Autodesk Fusion 360 part; units mm, degrees
sketch "Sketch1" plane through (0, 0, 0) normal (0, 0, 1) x (1, 0, 0)
  line L0 (13, -20) -> (-13, -20)
  line L1 (-13, -20) -> (-13, 20)
  line L2 (-13, 20) -> (13, 20)
  line L3 (13, 20) -> (13, -20)
  line L4 (13, -20) -> (-13, 20) construction
  line L5 (-13, -20) -> (13, 20) construction
  line L6 (0, 20) -> (0, -20)
  circle A0 centre (0, -4) radius 7
  circle A1 centre (0, 10) radius 1.7
  circle A2 centre (0, 10) radius 3
  line L7 (-3.85, 20) -> (-3.85, -20)
  line L8 (3.85, 20) -> (3.85, -20)
  circle A3 centre (0, -4) radius 1.7
  circle A4 centre (0, -4) radius 2.3
  line L9 (-3.85, 15) -> (3.85, 15)
  line L10 (-3.85, 5) -> (3.85, 5)
  line L11 (-3.85, -12) -> (3.85, -12)
  dimension "d1" = 26
  dimension "d2" = 40
  dimension "d3" = 14
  dimension "d4" = 16
  dimension "d5" = 3.4
  dimension "d6" = 6
  dimension "d7" = 7.7
  dimension "d8" = 10
  dimension "d9" = 3.4
  dimension "d10" = 4.6
  dimension "d15" = 5
  dimension "d16" = 5
  dimension "d17" = 8
extrude "Extrude1" add sketch "Sketch1" along normal blind 5 contours L0 L2 L3 A0 L8 | L0 L6 L8 L11 | L0 L6 L7 L11 | L6 A0 L8 L11 | L2 L6 L8 L9 | L0 L1 L2 A0 L7 | L6 A0 L7 L11 | A0 L8 | L6 A0 L8 A4 | L2 L6 L7 L9 | L6 A2 L8 L9 L10 | L6 A0 L7 A4 | L6 A0 L8 L10 | L6 A2 L7 L9 L10 | A0 L7 | L6 A3 A4 | L6 A3 A4 | L6 A0 L7 L10 | L6 A1 A2 | L6 A1 A2
extrude "Extrude13" cut sketch "Sketch1" along normal blind 10 contours L6 A3 | L6 A3 | L6 A1 | L6 A1
extrude "Extrude2" add sketch "Sketch1" along normal blind 0.8 from surface at 5 contours L0 L6 L8 L11 | L0 L6 L7 L11 | L2 L6 L8 L9 | L2 L6 L7 L9
fillet "Fillet1" radius 1 8 edges at (-3.85, 20, 5.4) (-3.85, 15, 5.4) (-3.85, -12, 5.4) (-3.85, -20, 5.4) (3.85, -12, 5.4) (3.85, -20, 5.4) (3.85, 15, 5.4) (3.85, 20, 5.4)
chamfer "Chamfer1" distance 0.2 angle 45 16 edges at (3.5571, 15.2929, 5.8) (0, 15, 5.8) (-3.5571, 15.2929, 5.8) (-3.85, 17.5, 5.8) (-3.5571, 19.7071, 5.8) (0, 20, 5.8) (3.5571, 19.7071, 5.8) (3.85, 17.5, 5.8) (3.5571, -19.7071, 5.8) (0, -20, 5.8) (-3.5571, -19.7071, 5.8) (-3.85, -16, 5.8) (-3.5571, -12.2929, 5.8) (0, -12, 5.8) (3.5571, -12.2929, 5.8) (3.85, -16, 5.8)
extrude "Extrude3" cut sketch "Sketch1" along normal blind 3 contours L6 A1 A2 | L6 A1 A2 | L6 A1 | L6 A1
extrude "Extrude5" cut sketch "Sketch1" against normal blind 5 from surface at 5 contours L6 A3 A4 | L6 A3 A4
chamfer "Chamfer3" distance 4 angle 45 4 edges at (13, -20, 2.5) (-13, -20, 2.5) (-13, 20, 2.5) (13, 20, 2.5)
fillet "Fillet2" radius 2 8 edges at (9, -20, 2.5) (-13, 16, 2.5) (13, -16, 2.5) (13, 16, 2.5) (9, 20, 2.5) (-9, 20, 2.5) (-13, -16, 2.5) (-9, -20, 2.5)
chamfer "Chamfer4" distance 0.2 angle 45 20 edges at (-2.1444, -3.1683, 5) (11, 18, 5) (8.9369, 19.8478, 5) (5.5108, 20, 5) (5.5108, -20, 5) (8.9369, -19.8478, 5) (11, -18, 5) (12.8478, -15.9369, 5) (13, 0, 5) (12.8478, 15.9369, 5) (-11, 18, 5) (-12.8478, 15.9369, 5) (-13, 0, 5) (-12.8478, -15.9369, 5) (-11, -18, 5) (-8.9369, -19.8478, 5) (-5.5108, -20, 5) (-5.5108, 20, 5) (-8.9369, 19.8478, 5) (-1.585, 10.6147, 5)
chamfer "Chamfer5" distance 1.5 angle 60 16 edges at (13, 0, 0) (12.8478, -15.9369, 0) (11, -18, 0) (8.9369, -19.8478, 0) (0, -20, 0) (-8.9369, -19.8478, 0) (-11, -18, 0) (-12.8478, -15.9369, 0) (-13, 0, 0) (-12.8478, 15.9369, 0) (-11, 18, 0) (-8.9369, 19.8478, 0) (0, 20, 0) (8.9369, 19.8478, 0) (11, 18, 0) (12.8478, 15.9369, 0) measured on face at (9.4248, -1.2191, 0) measured on face at (12.5321, -16.4571, 1.6) measured on face at (10.5286, -18.4714, 3.2) measured on face at (8.6045, -19.9526, 1.6) measured on face at (9.4248, -1.2191, 0) measured on face at (-9.4571, -19.5321, 1.6) measured on face at (-10.5286, -18.4714, 3.2) measured on face at (-12.6383, -16.3187, 3.2) measured on face at (9.4248, -1.2191, 0) measured on face at (-12.774, 16.0951, 1.6) measured on face at (-10.5286, 18.4714, 3.2) measured on face at (-9.4571, 19.5321, 3.2) measured on face at (9.4248, -1.2191, 0) measured on face at (9.0168, 19.8126, 1.6) measured on face at (11.4714, 17.5286, 3.2) measured on face at (12.8794, 15.8556, 1.6)
chamfer "Chamfer6" distance 0.4 angle 45 2 edges at (-2.797, 8.9152, 0) (-2.1444, -4.8317, 0) measured on face at (0.0573, -14.4312, 0) measured on face at (0.0573, -14.4312, 0)
sketch "Sketch11" plane through (0, 0, 3) normal (0, 0, -1) x (-1, 0, 0)
  circle A0 centre (0, 10) radius 1.7 construction
  circle A1 centre (0, 10) radius 3
  line L0 (0, 10) -> (1, 10) construction
  line L1 (-2.4712, 8.299) -> (2.4712, 8.299)
  line L2 (-2.4712, 11.701) -> (2.4712, 11.701)
  line L3 (0, 10) -> (0, 8.299) construction
  line L4 (0, 10) -> (0, 11.701) construction
  dimension "d87" = 1.701
  dimension "d88" = 1.701
extrude "Extrude16" cut sketch "Sketch11" against normal blind 0.2 contours A1 L1 L2
sketch "Sketch12" plane through (0, 0, 3.2) normal (0, 0, -1) x (-1, 0, 0)
  circle A0 centre (0, 10) radius 1.7 construction
  line L0 (-2.4712, 8.299) -> (2.4712, 8.299)
  arc A1 (2.4712, 8.299) -> (2.4712, 11.701) centre (0, 10) ccw
  line L1 (2.4712, 11.701) -> (-2.4712, 11.701)
  arc A2 (-2.4712, 11.701) -> (-2.4712, 8.299) centre (0, 10) ccw
  line L2 (0, 10) -> (1, 10) construction
  line L3 (0, 10) -> (0, 11) construction
  line L4 (1.701, 8.299) -> (1.701, 11.701)
  line L5 (-1.701, 8.299) -> (-1.701, 11.701)
  line L6 (0, 10) -> (1.701, 10) construction
  line L7 (0, 10) -> (-1.701, 10) construction
  dimension "d91" = 90
  dimension "d92" = 1.701
  dimension "d93" = 1.701
extrude "Extrude17" cut sketch "Sketch12" against normal blind 0.2 contours L0 L1 L4 L5
equation "d1 = 30 mm - 4 mm"
equation "d2 = 30 mm + 10 mm"
equation "d7 = 8 mm - 0.3 mm"
equation "d16 = d15"
equation "d17 = ( d3 / 2 ) + 1 mm"
Verification items for the finished model (mm, model axes). A direction names the side the tool comes from. Give positions to 0.01 mm unless a question says otherwise; leave off trailing zeros. Write each loop counter-clockwise with the first axis right and the second up, starting at its lowest first coordinate (ties: lowest second). Pieces come first, ordered by that corner, then holes. Notation, with made-up numbers: M 36,25.5 L 79,25.5 A18 cw 79,55.5 Z; hole C -39,71 d8. An arc over 180 degrees is marked long. One line per question, with ' | ' between items.
1) Mould release check, pull along Y, two halves, no side actions. Record for faces 1 (the flat face through (-11, -18, 4)), 2 (the flat face through (0, 12, 3)), 3 (the flat face through (0, 18, 5.8)): released by +Y, released by -Y, zero draft, split by the parting line, or undercut.
Result:
face 1: released by -Y | face 2: undercut | face 3: zero draft
2) Gauge pin test, flat ends, axial feed: pin 1 Ø2 at (x, y) = (-6, -11) entering from +Z; pin 2 Ø0.5 at (y, z) = (-17.5, 5.5) entering from -X; pin 3 Ø2.5 at (x, y) = (0, 11) entering from -Z. Record the tip position at first contact, or that the pin passes through.
Result:
pin 1: stops at z = 5 | pin 2: stops at x = -3.85 | pin 3: stops at z = 3
3) Thickness scan on line 1 along Y through (x, z) = (0, 4.3); line 2 along X through (y, z) = (-4, 3.25); line 3 along Y through (x, z) = (-0.75, 2.5). Record the ranges inside material, lowest first. Write a range as [from, to].
Result:
line 1: y = [-20, -6.3], [-1.7, 8.3], [11.7, 20] | line 2: x = [-13, -2.3], [2.3, 13] | line 3: y = [-19.94, -6.17], [-1.83, 7.1], [12.9, 19.94]
4) Section check C-C on x = -6.5. Enter the section's corners in (y, z), plus the area to 3 significant figures.
Result:
outline: M -20,2.6 L -18.5,0 L 18.5,0 L 20,2.6 L 20,4.8 L 19.8,5 L -19.8,5 L -20,4.8 Z | area: 196 mm2
5) Section check A-A on y = -4. Enter the section's corners in (x, z), plus the area to 3 significant figures.
Result:
outline: M -13,2.6 L -11.5,0 L -2.7,0 L -2.3,0.4 L -2.3,4.8 L -2.5,5 L -12.8,5 L -13,4.8 Z; M 2.3,0.4 L 2.7,0 L 11.5,0 L 13,2.6 L 13,4.8 L 12.8,5 L 2.5,5 L 2.3,4.8 Z | area: 103 mm2
6) Section check B-B on y = 14. Enter the section's corners in (x, z).
Result:
outline: M -13,2.6 L -11.5,0 L 11.5,0 L 13,2.6 L 13,4.8 L 12.8,5 L -12.8,5 L -13,4.8 Z
7) Set-up check for faces 4 (the cylindrical face through (3.549, -19.715, 5.294)), 5 (the flat face through (0, 8, 3)), 6 (the flat face through (12.26, 0.21, 1.32)): record each of +Z, -Z, +X, -X, +Y, -Y from which the full face is reachable in a straight line by a thin tool's end or side.
Result:
face 4: +Z, +X, -Y | face 5: -Z | face 6: -Z, +X, +Y, -Y
8) Section check D-D on z = 2.1. Enter the section's corners in (x, y).
Result:
outline: M -12.71,-15.17 A1.71 ccw -12.21,-16.38 L -9.38,-19.21 A1.71 ccw -8.17,-19.71 L 8.17,-19.71 A1.71 ccw 9.38,-19.21 L 12.21,-16.38 A1.71 ccw 12.71,-15.17 L 12.71,15.17 A1.71 ccw 12.21,16.38 L 9.38,19.21 A1.71 ccw 8.17,19.71 L -8.17,19.71 A1.71 ccw -9.38,19.21 L -12.21,16.38 A1.71 ccw -12.71,15.17 Z; hole C 0,10 d6; hole C 0,-4 d4.6
